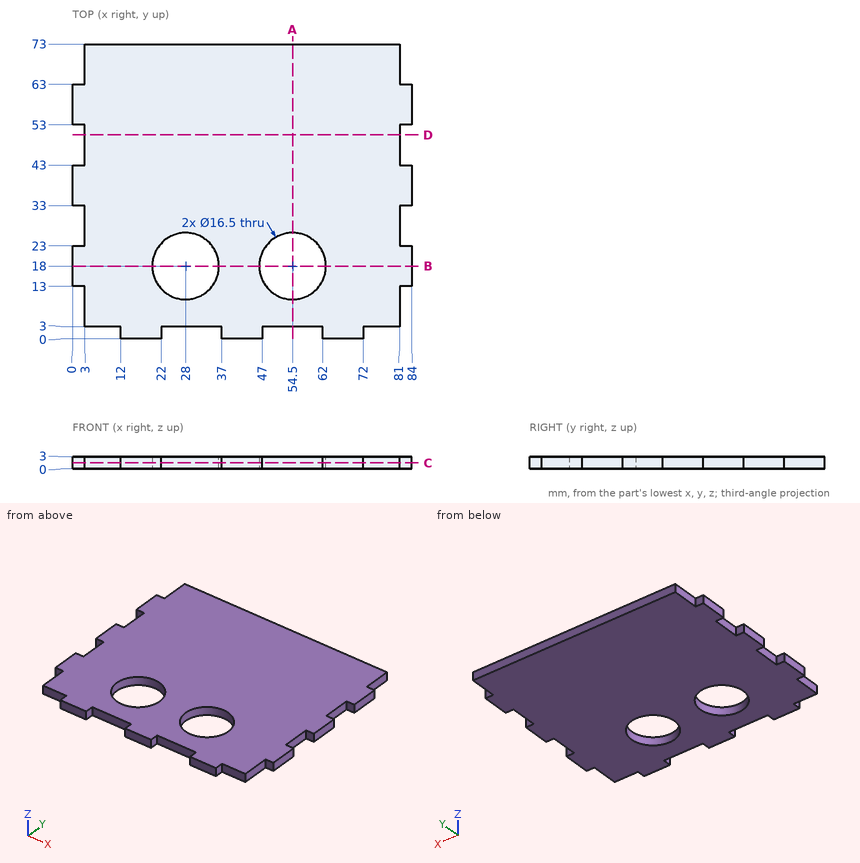
Geometry check sheet. Reference: drawing and pictorial views, mm from the part's lowest x, y, z. Give positions to 0.01 mm unless a question says otherwise; leave off trailing zeros. Write each loop counter-clockwise with the first axis right and the second up, starting at its lowest first coordinate (ties: lowest second). Pieces come first, ordered by that corner, then holes. Notation, with made-up numbers: (28.5, -18.75) -> (37.5, -18.75) arc R26 ccw to (37.5, 14.25) -> close; hole circle Ø9 at (8.25, 13.5). An arc over 180 degrees is marked (long way). One line per item, written item: value. Start each with the question number.
Item 1: Section check B-B on y = 18. Record the cut outline in (x, z).
Item 2: Section check C-C on z = 1.5. State how many separate pieces and enclosed holes the cut face has, then the cut area to 3 significant figures.
Item 3: Gauge pin test, flat ends, axial feed: pin 1 (1.5 mm diameter, centred on y = 8, z = 1, fed in from -X); pin 2 (1.5 mm diameter, centred on x = 82, z = 1, fed in from -Y); pin 3 (1.5 mm diameter, centred on x = 82.5, z = 1, fed in from +Y). Record the tip position at first contact, or that the pin passes through.
Item 4: Section check D-D on y = 50.5. Record the cut outline in (x, z), then the cut area to 3 significant figures.
Item 5: Section check A-A on x = 54.5. Record the cut outline in (y, z), then the cut area to 4 significant figures.
Item 6: Material ranges on probe 1 along Y at (x, z) = (28, 2.2); probe 2 along X at (y, z) = (24.5, 2.7); probe 3 along X at (y, z) = (47, 1.65), recorded low to high. Write a range as from..to.
Results list:
1. outline: (0, 0) -> (19.75, 0) -> (19.75, 3) -> (0, 3) -> close; (36.25, 0) -> (46.25, 0) -> (46.25, 3) -> (36.25, 3) -> close; (62.75, 0) -> (84, 0) -> (84, 3) -> (62.75, 3) -> close
2. separate pieces: 1
2. enclosed holes: 2
2. area: 5,300 mm²
3. pin 1: x = 3
3. pin 2: y = 13
3. pin 3: y = 63
4. outline: (3, 0) -> (81, 0) -> (81, 3) -> (3, 3) -> close
4. area: 234 mm²
5. outline: (3, 0) -> (9.75, 0) -> (9.75, 3) -> (3, 3) -> close; (26.25, 0) -> (73, 0) -> (73, 3) -> (26.25, 3) -> close
5. area: 160.5 mm²
6. probe 1: 3..9.75, 26.25..73
6. probe 2: 3..22.92, 33.08..49.42, 59.58..81
6. probe 3: 3..81
